Could you check a few things on this model? Use its own coordinates, in mm. A direction names the side the tool comes from. Round coordinates to 2 decimals unless told otherwise and drop trailing zeros. Order: outer loops, then holes, each group sorted by start corner. A loop starts at its lowest first (then second) coordinate and runs counter-clockwise, first axis right, second up. Notation, with made-up numbers: (2, 34) - (45, 34) arc R22 ccw to (45, 46) - close; hole circle Ø4 at (45, 49). An arc over 180 degrees is marked (long way). Return JSON: item names as keys, results as strings. Group by question number.
from build123d import *

# Parameters (mm, degrees)
SKETCH1_R                  = 35
BOSS_EXTRUDE1_DEPTH        = 7
SKETCH2_R                  = 17.5
CUT_EXTRUDE1_DEPTH         = 50.989999
CIRPATTERN1_COUNT          = 6
F_10_0_10_DIAMETER_HOLE1_D = 10
LPATTERN1_COUNT            = 2
LPATTERN1_PITCH            = 23
LPATTERN1_COUNT_DIR2       = 2
LPATTERN1_PITCH_DIR2       = 40
CUT_EXTRUDE2_DEPTH         = 49.413170413
SKETCH11_W                 = 15
SKETCH11_H                 = 8
BOSS_EXTRUDE2_DEPTH        = 22
FILLET1_RADIUS             = 7.5
FILLET1_LENGTH             = 8
M10_TAPPED_HOLE1_D         = 8.5
FILLET2_R                  = 2


with BuildPart() as part:
    # Sketch1 → Boss-Extrude1 (new body)
    with BuildSketch(Plane(origin=(0, 0, 0), x_dir=(1, 0, 0), z_dir=(0, 1, 0))):
        with Locations(Location((0, 0, 0), (0, 0, 270))):
            Circle(SKETCH1_R)
    extrude(amount=BOSS_EXTRUDE1_DEPTH)

    # Sketch2 → Cut-Extrude1 (cut, through all)
    with BuildSketch(Plane(origin=(0, 7, 0), x_dir=(1, 0, 0), z_dir=(0, 1, 0))):
        with Locations((0, 45)):
            Circle(SKETCH2_R)
    cut_extrude1 = extrude(amount=-CUT_EXTRUDE1_DEPTH, mode=Mode.SUBTRACT)

    # CirPattern1: Cut-Extrude1 ×6 about axis
    cirpattern1_axis = Axis((0, 0, 0), (0, 1, 0))
    for i in range(1, CIRPATTERN1_COUNT):
        add(cut_extrude1.rotate(cirpattern1_axis, i * 360 / CIRPATTERN1_COUNT), mode=Mode.SUBTRACT)

    # Ø10.0 (10) Diameter Hole1 (through all)
    with Locations(Plane(origin=(0, 7, 0), x_dir=(1, 0, 0), z_dir=(0, 1, 0))):
        with Locations((-11.5, 20)):
            f_10_0_10_diameter_hole1 = Hole(F_10_0_10_DIAMETER_HOLE1_D / 2)

    # LPattern1: 10.0 _10_ Diameter Hole1 2 × 2
    with Locations(*[(i * LPATTERN1_PITCH, 0, j * LPATTERN1_PITCH_DIR2) for i in range(LPATTERN1_COUNT) for j in range(LPATTERN1_COUNT_DIR2) if (i, j) != (0, 0)]):
        add(f_10_0_10_diameter_hole1, mode=Mode.SUBTRACT)

    # Sketch9 → Cut-Extrude2 (cut, through all)
    with BuildSketch(Plane(origin=(0, 7, 0), x_dir=(1, 0, 0), z_dir=(0, 1, 0))):
        with BuildLine():
            Line((12.990381057, -7.5), (19.485571585, -11.25))
            ThreePointArc((19.485571585, -11.25), (23.964805416, -5.735160985), (29.940285542, -1.891904249))
            ThreePointArc((29.940285542, -1.891904249), (30, 0), (29.940285542, 1.891904249))
            ThreePointArc((29.940285542, 1.891904249), (23.964805416, 5.735160985), (19.485571585, 11.25))
            Line((19.485571585, 11.25), (12.990381057, 7.5))
            ThreePointArc((12.990381057, 7.5), (15, 0), (12.990381057, -7.5))
        make_face()
    cut_extrude2 = extrude(amount=-CUT_EXTRUDE2_DEPTH, mode=Mode.SUBTRACT)

    # Mirror1: Cut-Extrude2 across plane
    add(cut_extrude2.mirror(Plane(origin=(0, 0, 0), x_dir=(0, 0, 1), z_dir=(1, 0, 0))), mode=Mode.SUBTRACT)

    # Sketch11 → Boss-Extrude2 (add)
    with BuildSketch(Plane(origin=(0, 0, 0), x_dir=(1, 0, 0), z_dir=(0, 1, 0))):
        Rectangle(SKETCH11_W, SKETCH11_H)
    extrude(amount=BOSS_EXTRUDE2_DEPTH)

    # Fillet1: full round fillet: the end face becomes a half cylinder, R = half its width
    fillet1_face = Plane((0, 22, 0), x_dir=(0, 0, -1), z_dir=(0, 1, 0))  # on the end face: x along it, z out of the body
    fillet1_slab = fillet1_face.offset(-FILLET1_RADIUS / 2) * Box(FILLET1_LENGTH, 2 * FILLET1_RADIUS, FILLET1_RADIUS, mode=Mode.PRIVATE)  # the body's end, R deep
    fillet1_round = Plane((0, 14.5, 0), x_dir=(0, 1, 0), z_dir=(0, 0, -1)) * Cylinder(FILLET1_RADIUS, FILLET1_LENGTH, mode=Mode.PRIVATE)  # its axis R under the face
    add(fillet1_slab - fillet1_round, mode=Mode.SUBTRACT)

    # M10 Tapped Hole1 (through all)
    with Locations(Plane.XY.offset(4)):
        with Locations((0, 14.5)):
            Hole(M10_TAPPED_HOLE1_D / 2)

    # Fillet2
    fillet2_edges = [part.edges().sort_by_distance(p)[0] for p in [
        (7.5, 7, 0),
        (-7.5, 7, 0),
    ]]
    fillet(fillet2_edges, radius=FILLET2_R)


solid = part.part
1) Will these pins go through, and if not, where does the flat tip stop? pin 1 (4.5 mm diameter, centred on x = 1, y = 15.5, fed in from -Z); pin 2 (5 mm diameter, centred on y = 2.5, z = 18.5, fed in from -X); pin 3 (3 mm diameter, centred on y = 6.5, z = -11, fed in from -X); pin 4 (3 mm diameter, centred on y = 18.5, z = 3, fed in from -X).
2) We'd pull the mould along Z, two halves only. Please class faces 1 (the cylindrical face through (35, 3, 0)), 2 (the cylindrical face through (-23.72, 3.55, 13.92)), 3 (the flat face through (0, 9, -4)): +Z half, -Z half, draft (parallel to the pull), parting line (faces both ways), or undercut.
3) I want a section at D-D, the plane y = 15.5. List the corners of the cut face in (x, z) for me.
4) I want a section at C-C, the plane x = 11.5. List the corners of the cut face in (y, z) for me, plus the area to 3 significant figures.
5) For faces 4 (the flat face through (0, 9, 4)), 5 (the cylindrical face through (17.43, 3.45, 30.35)), 6 (the cylindrical face through (-0.2, 3.5, -27.5)), 7 (the flat face through (7.5, 12, 0)), 8 (the cylindrical face through (-24.04, 3.55, -5.67)), which set-ups out of +Z, -Z, +X, -X, +Y, -Y let a thin tool reach every point of the face, with its end or its side?
6) I want a section at B-B, the plane z = -9. List the corners of the cut face in (x, y) for me, plus the area to 3 significant figures.
7) I want a section at A-A, the plane x = 0. List the corners of the cut face in (y, z) for me.
8) If I drill on line 1 along Y through (x, z) = (0, -0.75); line 2 along Z through (x, y) = (-11.5, 2.5); line 3 along Y through (x, z) = (-7, 26), over which ranges is the centre line in solid material (lowest first)? Write a range as from..to.
Outcome:
{
 "1": {"pin 1": "through", "pin 2": "x = -22.72", "pin 3": "x = -27.26", "pin 4": "x = -7.07"},
 "2": {"face 1": "parting line", "face 2": "undercut", "face 3": "-Z half"},
 "3": {"outline": "(-7.43, -4) - (-4.13, -4) - (-4.13, 4) - (-7.43, 4) - close; (4.13, -4) - (7.43, -4) - (7.43, 4) - (4.13, 4) - close"},
 "4": {"outline": "(0, -31.81) - (7, -31.81) - (7, -25) - (0, -25) - close; (0, -15) - (7, -15) - (7, 15) - (0, 15) - close; (0, 25) - (7, 25) - (7, 31.81) - (0, 31.81) - close", "area": "305 mm^2"},
 "5": {"face 4": "+Z, +X, -X, +Y", "face 5": "+Z, +X, +Y, -Y", "face 6": "-Z, +Y, -Y", "face 7": "+Z, -Z, +X, +Y", "face 8": "+Y, -Y"},
 "6": {"outline": "(-27.84, 0) - (-20.97, 0) - (-20.97, 7) - (-27.84, 7) - close; (-15.59, 0) - (15.59, 0) - (15.59, 7) - (-15.59, 7) - close; (20.97, 0) - (27.84, 0) - (27.84, 7) - (20.97, 7) - close", "area": "314 mm^2"},
 "7": {"outline": "(0, -27.5) - (7, -27.5) - (7, -4) - (10.25, -4) - (10.25, 4) - (7, 4) - (7, 27.5) - (0, 27.5) - close; (18.75, -4) - (22, -4) - (22, 4) - (18.75, 4) - close"},
 "8": {"line 1": "0..10.25, 18.75..22", "line 2": "-31.81..-25, -15..15, 25..31.81", "line 3": "0..7"}
}
